Work out the finished part from the listing and answer in its coordinate system (mm). Face numbers are marked on the shaded views. A direction names the side the tool comes from. Give positions to 0.01 mm unless a question says otherwise; leave off trailing zeros. Write each loop counter-clockwise with the first axis right and the second up, starting at its lowest first coordinate (ties: lowest second). Pieces come first, ordered by that corner, then holes. Notation, with made-up numbers: (-18.5, 23.5) -> (38.5, 23.5) arc R18 ccw to (38.5, 43.5) -> close; hole circle Ø10 at (-39, -19.5). An arc over 180 degrees is marked (long way). Use a Markdown table: item, result. Add a question column.
Q1. Each of these flat-tipped pins is pushed along its axis until it touches: pin 1 Ø6 at (x, z) = (28.5, -13.5) entering from +Y; pin 2 Ø6 at (x, y) = (25.5, 52) entering from +Z (3 decimals); pin 3 Ø7 at (x, y) = (17.5, 49.5) entering from -Z (3 decimals). Where does it stop, or does it pass through?
Q2. Section A-A, the plane x = 42 is taken. Give the vertices of the cut face in (y, z) (3 decimals), plus the area to 3 significant figures.
Q3. Section C-C, the plane z = -16.5 is taken. Give the vertices of the cut face in (x, y), plus the area to 3 significant figures.
Q4. Consider line 1 (Z direction, x = 13.5, y = 52) (3 decimals); line 2 (Z direction, x = 3, y = 29.5); line 3 (Y direction, x = 44, z = -61). Determine where each line is inside the solid, lowest interval first.
Q5. For a pull along Z with two mould halves and no side action, classify the marked faces 1, 2 and 3 as pulls with the +Z half, pulls with the -Z half, needs draft (parallel to the pull), parting line crosses it, or undercut.
Q6. Section B-B, the plane y = 51.5 is taken. Give the vertices of the cut face in (x, z) (3 decimals).
Q7. For the marked faces 4 and 5, determine the directions among +Z, -Z, +X, -X, +Y, -Y from which every point of the face is accessible in a straight line to the end or side of a thin tool.
from build123d import *

# Parameters (mm, degrees)
SKETCH_1_W          = 52.5
SKETCH_1_H          = 90
EXTRUDE_1_DEPTH     = 58.4
SKETCH_3_W          = 52.5
SKETCH_3_H          = 22.425
CUT_EXTRUDE_1_DEPTH = 15
SKETCH_4_W          = 52.5
SKETCH_4_H          = 13.18
SKETCH_4_H_2        = 13.17
CUT_EXTRUDE_2_DEPTH = 15
CHAMFER_1_SIZE      = 5
SKETCH_5_W          = 52.5
SKETCH_5_H          = 36
CUT_EXTRUDE_3_DEPTH = 3.9
FILLET_1_R          = 1


with BuildPart() as part:
    # Эскиз1 → Бобышка-Вытянуть1 (new body)
    with BuildSketch(Plane(origin=(0, 0, 0), x_dir=(1, 0, 0), z_dir=(0, 1, 0))):
        with Locations((26.25, 45)):
            Rectangle(SKETCH_1_W, SKETCH_1_H)
    extrude(amount=EXTRUDE_1_DEPTH)

    # Эскиз3 → Вырез-Вытянуть1 (cut)
    with BuildSketch(Plane(origin=(0, 58.4, 0), x_dir=(1, 0, 0), z_dir=(0, 1, 0))):
        with Locations((26.25, 78.7875)):
            Rectangle(SKETCH_3_W, SKETCH_3_H)
        with Locations((26.25, 11.2125)):
            Rectangle(SKETCH_3_W, SKETCH_3_H)
    extrude(amount=-CUT_EXTRUDE_1_DEPTH, mode=Mode.SUBTRACT)

    # Эскиз4 → Вырез-Вытянуть2 (cut)
    with BuildSketch(Plane(origin=(0, 43.4, 0), x_dir=(1, 0, 0), z_dir=(0, 1, 0))):
        with Locations((26.25, 83.41)):
            Rectangle(SKETCH_4_W, SKETCH_4_H)
        with Locations((26.25, 6.585)):
            Rectangle(SKETCH_4_W, SKETCH_4_H_2)
    extrude(amount=-CUT_EXTRUDE_2_DEPTH, mode=Mode.SUBTRACT)

    # Фаска1
    chamfer_1_edges = [part.edges().sort_by_distance(p)[0] for p in [
        (26.25, 58.4, -67.575),
        (26.25, 58.4, -22.425),
    ]]
    chamfer(chamfer_1_edges, length=CHAMFER_1_SIZE)

    # Эскиз5 → Вырез-Вытянуть3 (cut)
    with BuildSketch(Plane.XZ):
        with Locations((26.25, -45)):
            Rectangle(SKETCH_5_W, SKETCH_5_H)
    extrude(amount=-CUT_EXTRUDE_3_DEPTH, mode=Mode.SUBTRACT)

    # Скругление1
    fillet_1_edges = [part.edges().sort_by_distance(p)[0] for p in [
        (26.25, 43.4, -67.575),
        (26.25, 43.4, -22.425),
        (26.25, 0, -90),
        (26.25, 28.4, -90),
        (26.25, 28.4, -76.82),
        (26.25, 43.4, -76.82),
        (26.25, 0, 0),
        (26.25, 28.4, -13.17),
        (26.25, 28.4, 0),
        (26.25, 43.4, -13.17),
    ]]
    fillet(fillet_1_edges, radius=FILLET_1_R)


solid = part.part
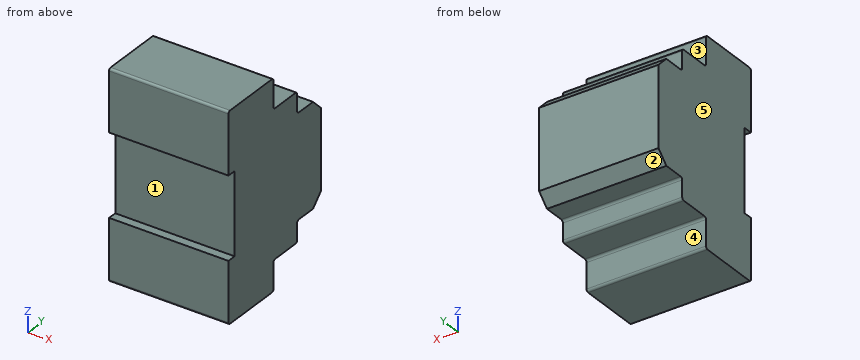
Result set:
| question | item | result |
|---|---|---|
| 1 | pin 1 | stops at y = 43.4 |
| 1 | pin 2 | stops at z = -22.425 |
| 1 | pin 3 | stops at z = -67.575 |
| 2 | outline | (0, -89) arc R1 ccw to (1, -90) -> (27.4, -90) arc R1 ccw to (28.4, -89) -> (28.4, -77.82) arc R1 cw to (29.4, -76.82) -> (42.4, -76.82) arc R1 ccw to (43.4, -75.82) -> (43.4, -68.575) arc R1 cw to (44.4, -67.575) -> (53.4, -67.575) -> (58.4, -62.575) -> (58.4, -27.425) -> (53.4, -22.425) -> (44.4, -22.425) arc R1 cw to (43.4, -21.425) -> (43.4, -14.17) arc R1 ccw to (42.4, -13.17) -> (29.4, -13.17) arc R1 cw to (28.4, -12.17) -> (28.4, -1) arc R1 ccw to (27.4, 0) -> (1, 0) arc R1 ccw to (0, -1) -> (0, -27) -> (3.9, -27) -> (3.9, -63) -> (0, -63) -> close |
| 2 | area | 4,020 mm2 |
| 3 | outline | (0, 0) -> (52.5, 0) -> (52.5, 43.4) -> (0, 43.4) -> close |
| 3 | area | 2,280 mm2 |
| 4 | line 1 | z = -67.575 to -22.425 |
| 4 | line 2 | z = -76.82 to -13.17 |
| 4 | line 3 | y = 3.9 to 58.4 |
| 5 | face 1 | undercut |
| 5 | face 2 | pulls with the -Z half |
| 5 | face 3 | needs draft |
| 6 | outline | (0, -67.575) -> (52.5, -67.575) -> (52.5, -22.425) -> (0, -22.425) -> close |
| 7 | face 4 | -Z, +X, -X, +Y |
| 7 | face 5 | +Z, -Z, -X, +Y, -Y |
